Input: part model. Units: mm. Frame: model coordinates. Face numbers are marked on the shaded views. A direction names the side the tool comes from. Round coordinates to 2 decimals unless told otherwise and drop trailing zeros. Order: outer loops, then holes, each group sorted by start corner. A loop starts at its lowest first (then second) coordinate and runs counter-clockwise, first axis right, second up. Notation, with made-up numbers: (-31, 53) - (-18, 53) arc R20 ccw to (-18, 83) - close; hole circle Ø4 at (79.5, 89.25). An arc over 180 degrees is marked (long way). One line per item, written item: value. Start each with the question number.
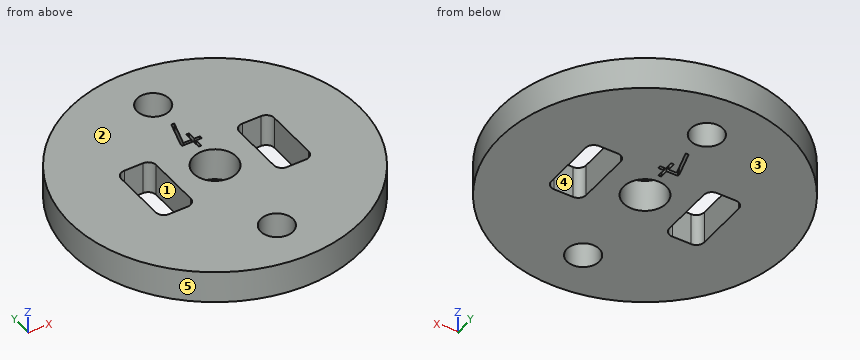
from build123d import *

# Parameters (mm, degrees)
MODEL_R                 = 13.5
MODEL_R_2               = 2
MODEL_R_3               = 1.5
SALIENTE_EXTRUIR1_DEPTH = 3


with BuildPart() as part:
    # Model → Saliente-Extruir1 (new body)
    with BuildSketch(Plane.XY):
        with Locations((21.167864369, 286.142389673)):
            Circle(MODEL_R)
        with Locations((21.167864369, 286.142389673)):
            Circle(MODEL_R_2, mode=Mode.SUBTRACT)
        with Locations((21.167864369, 295.142389673)):
            Circle(MODEL_R_3, mode=Mode.SUBTRACT)
        with Locations((21.167864369, 277.142389673)):
            Circle(MODEL_R_3, mode=Mode.SUBTRACT)
        with BuildLine():
            Line((27.542864369, 289.392389673), (25.792864369, 289.392389673))
            ThreePointArc((25.792864369, 289.392389673), (25.262534283, 289.172719759), (25.042864369, 288.642389673))
            Line((25.042864369, 288.642389673), (25.042864369, 283.642389673))
            ThreePointArc((25.042864369, 283.642389673), (25.262534283, 283.112059587), (25.792864369, 282.892389673))
            Line((25.792864369, 282.892389673), (27.542864369, 282.892389673))
            ThreePointArc((27.542864369, 282.892389673), (28.073194454, 283.112059587), (28.292864369, 283.642389673))
            Line((28.292864369, 283.642389673), (28.292864369, 288.642389673))
            ThreePointArc((28.292864369, 288.642389673), (28.073194454, 289.172719759), (27.542864369, 289.392389673))
        make_face(mode=Mode.SUBTRACT)
        with BuildLine():
            Line((14.792864369, 289.392389673), (16.542864369, 289.392389673))
            ThreePointArc((16.542864369, 289.392389673), (17.073194454, 289.172719759), (17.292864369, 288.642389673))
            Line((17.292864369, 288.642389673), (17.292864369, 283.642389673))
            ThreePointArc((17.292864369, 283.642389673), (17.073194454, 283.112059587), (16.542864369, 282.892389673))
            Line((16.542864369, 282.892389673), (14.792864369, 282.892389673))
            ThreePointArc((14.792864369, 282.892389673), (14.262534283, 283.112059587), (14.042864369, 283.642389673))
            Line((14.042864369, 283.642389673), (14.042864369, 288.642389673))
            ThreePointArc((14.042864369, 288.642389673), (14.262534283, 289.172719759), (14.792864369, 289.392389673))
        make_face(mode=Mode.SUBTRACT)
        Polygon((22.128307957, 289.571683654), (21.605919898, 289.571683654), (21.605919898, 288.788101564), (21.344725868, 288.788101564), (21.344725868, 289.571683654), (20.299949748, 289.571683654), (20.299949748, 289.804309587), (21.032925495, 292.288101564), (21.303914301, 292.283204176), (20.577468405, 289.832877684), (21.344725868, 289.832877684), (21.344725868, 290.616459773), (21.605919898, 290.616459773), (21.605919898, 289.832877684), (22.128307957, 289.832877684), align=None, mode=Mode.SUBTRACT)
    extrude(amount=SALIENTE_EXTRUIR1_DEPTH)


solid = part.part
Item 1: First-contact query: pin 1 Ø0.6 at (y, z) = (290.5, 2) entering from -X; pin 2 Ø3.5 at (x, y) = (21.17, 286.14) entering from +Z; pin 3 Ø0.5 at (x, z) = (15.5, 1.5) entering from -Y; pin 4 Ø0.9 at (x, z) = (26.5, 2) entering from +Y. Flat tips, straight axial feed; report the tip coordinate or a pass-through.
Item 2: Section query C-C on z = 2.55. Give the number of separate pieces and of enclosed holes in the cut face, and give its area (3 significant figures).
Item 3: Section query B-B on y = 295.5. Return loops of the section in (x, z), and give its area (3 significant figures).
Item 4: Reachability of the marked faces 1 and 2 from +Z, -Z, +X, -X, +Y, -Y: full face, straight path, thin tool, end or side. Return the list, or none.
Item 5: Section query A-A on x = 16. Return loops of the section in (y, z).
Item 6: Section query D-D on x = 11. Return loops of the section in (y, z), and give its area (3 significant figures).
Item 7: Pull-direction query (X, two-part tool) for the marked faces 3, 4 and 5; classes: released by +X, released by -X, zero draft, split by the parting line, or undercut.
Item 8: Line query: L1, parallel to X at y = 288.5, z = 2.2; L2, parallel to Y at x = 22, z = 2.65; L3, parallel to X at y = 283.5, z = 1.35. Output: solid intervals per line, ascending.
Geometry results:
1. pin 1: stops at x = 8.29
1. pin 2: passes through
1. pin 3: stops at y = 273.78
1. pin 4: stops at y = 298.73
2. separate pieces: 1
2. enclosed holes: 6
2. area: 503 mm^2
3. outline: (11.44, 0) - (19.71, 0) - (19.71, 3) - (11.44, 3) - close; (22.62, 0) - (30.9, 0) - (30.9, 3) - (22.62, 3) - close
3. area: 49.6 mm^2
4. face 1: +Z, -Z
4. face 2: +Z, +X, -X, +Y, -Y
5. outline: (273.67, 0) - (282.89, 0) - (282.89, 3) - (273.67, 3) - close; (289.39, 0) - (298.61, 0) - (298.61, 3) - (289.39, 3) - close
6. outline: (277.26, 0) - (295.02, 0) - (295.02, 3) - (277.26, 3) - close
6. area: 53.3 mm^2
7. face 3: zero draft
7. face 4: undercut
7. face 5: split by the parting line
8. L1: x = 7.88 to 14.04, 17.29 to 25.04, 28.29 to 34.46
8. L2: y = 272.67 to 275.89, 278.39 to 284.32, 287.96 to 289.57, 289.83 to 293.89, 296.39 to 299.62
8. L3: x = 7.93 to 14.06, 17.28 to 25.06, 28.28 to 34.41
